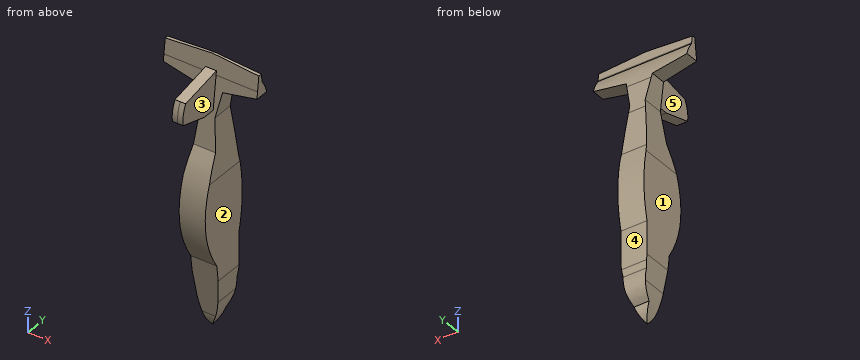
```python
from build123d import *

# Parameters (mm, degrees)
BOSS_EXTRUDE1_DEPTH      = 240
SKETCH4_OUTSIDE_W        = 620.683
SKETCH4_OUTSIDE_H        = 358.674
CUT_EXTRUDE1_DEPTH       = 251.005507708
BOSS_EXTRUDE2_DEPTH      = 10
BOSS_EXTRUDE2_DEPTH_BACK = 10


with BuildPart() as part:
    # Sketch3 → Boss-Extrude1 (new body)
    with BuildSketch(Plane(origin=(0, 0, 0), x_dir=(1, 0, 0), z_dir=(0, 1, 0))):
        with BuildLine():
            Line((137.970364324, 414.272883639), (137.970364324, 223.69340993))
            add(Edge.make_bspline(
                [(137.970364324, 223.69340993), (141.476966078, 171.478024708), (148.044741181, 119.610332165)],
                knots=[0, 0, 0, 0.887153435, 0.887153435, 0.887153435], degree=2))
            Line((148.044741181, 119.610332165), (137.970364324, 72.071329968))
            Line((137.970364324, 72.071329968), (74.77736212, 59.754974694))
            Line((74.77736212, 59.754974694), (74.77736212, 19.446902889))
            Line((74.77736212, 19.446902889), (162.391434864, 12.728890921))
            Line((162.391434864, 12.728890921), (250.005507608, 19.446902889))
            Line((250.005507608, 19.446902889), (250.005507608, 59.754974694))
            Line((250.005507608, 59.754974694), (186.812505404, 72.071329968))
            Line((186.812505404, 72.071329968), (176.738128547, 119.610332165))
            add(Edge.make_bspline(
                [(186.812505404, 223.69340993), (183.30590365, 171.478024708), (176.738128547, 119.610332165)],
                knots=[0, 0, 0, 0.887153435, 0.887153435, 0.887153435], degree=2))
            Line((186.812505404, 223.69340993), (186.812505404, 414.272883639))
            Line((186.812505404, 414.272883639), (182.139885098, 458.943511131))
            add(Edge.make_bspline(
                [(182.139885098, 458.943511131), (178.393317936, 491.021832881), (162.391434864, 514.737632441)],
                knots=[0, 0, 0, 0.490132675, 0.490132675, 0.490132675], degree=2))
            add(Edge.make_bspline(
                [(142.64298463, 458.943511131), (146.389551792, 491.021832881), (162.391434864, 514.737632441)],
                knots=[0, 0, 0, 0.490132675, 0.490132675, 0.490132675], degree=2))
            Line((142.64298463, 458.943511131), (137.970364324, 414.272883639))
        make_face()
    extrude(amount=BOSS_EXTRUDE1_DEPTH)

    # Sketch4 outside → Cut-Extrude1 (cut, through all)
    with BuildSketch(Plane(origin=(0, 0, 0), x_dir=(0, 0, -1), z_dir=(1, 0, 0))):
        with Locations((263.7335, 120)):
            Rectangle(SKETCH4_OUTSIDE_W, SKETCH4_OUTSIDE_H)
        with BuildLine():
            Line((12.728890921, 85.924982425), (46.991957136, 81.651030623))
            Line((46.991957136, 81.651030623), (177.382016131, 65.386262487))
            add(Edge.make_bspline(
                [(177.382016131, 65.386262487), (287.640309593, 1.862307292), (384.386809277, 63.333754572)],
                knots=[0, 0, 0, 1, 1, 1], degree=2))
            Line((384.386809277, 63.333754572), (489.693965282, 76.663405275))
            add(Edge.make_bspline(
                [(489.693965282, 76.663405275), (505.317689733, 77.809278687), (514.737632441, 87.136419671)],
                knots=[0, 0, 0, 0.756426815, 0.756426815, 0.756426815], degree=2))
            add(Edge.make_bspline(
                [(514.737632441, 87.136419671), (501.382115592, 101.295387019), (485.88559641, 101.608221382)],
                knots=[0, 0, 0, 0.70811857, 0.70811857, 0.70811857], degree=2))
            add(Edge.make_bspline(
                [(485.88559641, 101.608221382), (473.943480605, 117.077174504), (457.892628594, 123.023372981), (437.733040377, 119.446816811)],
                knots=[0, 0, 0, 0, 0.856300563, 0.856300563, 0.856300563, 0.856300563], degree=3))
            Line((437.733040377, 119.446816811), (424.380439139, 121.602157956))
            Line((424.380439139, 121.602157956), (352.592685915, 121.602157956))
            add(Edge.make_bspline(
                [(352.592685915, 121.602157956), (283.160705497, 138.135189476), (211.297296684, 121.602157956)],
                knots=[0, 0, 0, 1, 1, 1], degree=2))
            Line((211.297296684, 121.602157956), (132.668959601, 113.79500177))
            Line((132.668959601, 113.79500177), (78.849169619, 108.45113311))
            add(Edge.make_bspline(
                [(78.849169619, 108.45113311), (52.309636156, 107.107843422), (34.577807776, 93.377447612)],
                knots=[0, 0, 0, 0.568417753, 0.568417753, 0.568417753], degree=2))
            Line((34.577807776, 93.377447612), (32.858632307, 93.377447612))
            Line((32.858632307, 93.377447612), (12.728890921, 90.430289665))
            Line((12.728890921, 90.430289665), (12.728890921, 85.924982425))
        make_face(mode=Mode.SUBTRACT)
    extrude(amount=CUT_EXTRUDE1_DEPTH, mode=Mode.SUBTRACT)

    # Sketch5 → Boss-Extrude2 (add, two sides)
    with BuildSketch(Plane.ZY.offset(-162.391434864)) as boss_extrude2_sk:
        with BuildLine():
            Line((-39.600938792, 82.572981273), (-55.527663258, 2.06573062))
            add(Edge.make_bspline(
                [(-55.527663258, 2.06573062), (-74.440482287, -7.393827092), (-92.263908139, -4.476340386)],
                knots=[0, 0, 0, 0.637969312, 0.637969312, 0.637969312], degree=2))
            Line((-92.263908139, -4.476340386), (-107.864231307, 50.87964505))
            Line((-107.864231307, 50.87964505), (-107.864231307, 74.057864143))
            Line((-107.864231307, 74.057864143), (-39.600938792, 82.572981273))
        make_face()
    extrude(amount=BOSS_EXTRUDE2_DEPTH)
    extrude(boss_extrude2_sk.sketch, amount=-BOSS_EXTRUDE2_DEPTH_BACK)


solid = part.part
```
Design review of the part built by this model. Coordinates are the model's own, in mm. Face numbers are marked on the shaded views. A direction names the side the tool comes from. Coordinates: 2 decimals unless noted, no trailing zeros. Order: outer loops, then holes, each group sorted by start corner. A loop starts at its lowest first (then second) coordinate and runs counter-clockwise, first axis right, second up. Notation, with made-up numbers: M -11.5,53 L 2.5,53 A25 ccw 2.5,84 Z; hole C 37,64 d7. An arc over 180 degrees is marked long. Answer as a JSON object with one key per item and string values. Group by question number.
1) Wall thickness on L1, parallel to X at y = 66, z = -52.5; L2, parallel to X at y = 109, z = -260.5; L3, parallel to Y at x = 156, z = -351: over which ranges is each line inside the solid? List them lowest first.
2) Add section A-A, the plane z = -98.5. Write out the cut boundary in (x, y), then the cut area to 3 significant figures.
3) For pin 1 (10 mm diameter, centred on y = 61.5, z = -182.5, fed in from +X); pin 2 (10 mm diameter, centred on y = 98.5, z = -119, fed in from +X); pin 3 (6 mm diameter, centred on y = 48, z = -221.5, fed in from +X), all flat-tipped, find the tip position at first contact; note any pin that passes through.
4) Tool access review of the marked faces 1, 2, 3, 4 and 5: name each direction out of +Z, -Z, +X, -X, +Y, -Y from which nothing blocks a thin tool from reaching the whole face with its end or side.
5) Add section B-B, the plane y = 12. Write out the cut boundary in (x, z), then the cut area to 3 significant figures.
Computed values:
{
 "1": {"L1": "x = 152.39 to 172.39", "L2": "x = 137.97 to 186.81", "L3": "y = 46 to 121.98"},
 "2": {"outline": "M 143.57,75.23 L 152.39,75.23 L 152.39,17.65 L 172.39,17.65 L 172.39,75.23 L 181.21,75.23 L 181.21,110.4 L 143.57,110.4 Z", "area": "2,480 mm^2"},
 "3": {"pin 1": "stops at x = 184.01", "pin 2": "stops at x = 177.93", "pin 3": "stops at x = 186.81"},
 "4": {"face 1": "-Z, -X, +Y, -Y", "face 2": "-Z, +X, +Y, -Y", "face 3": "+Z, +X, -Y", "face 4": "-Z, +X, -X, +Y", "face 5": "+Z, -X, -Y"},
 "5": {"outline": "M 152.39,-96.91 L 172.39,-96.91 L 172.39,-53.56 L 152.39,-53.56 Z", "area": "867 mm^2"}
}
